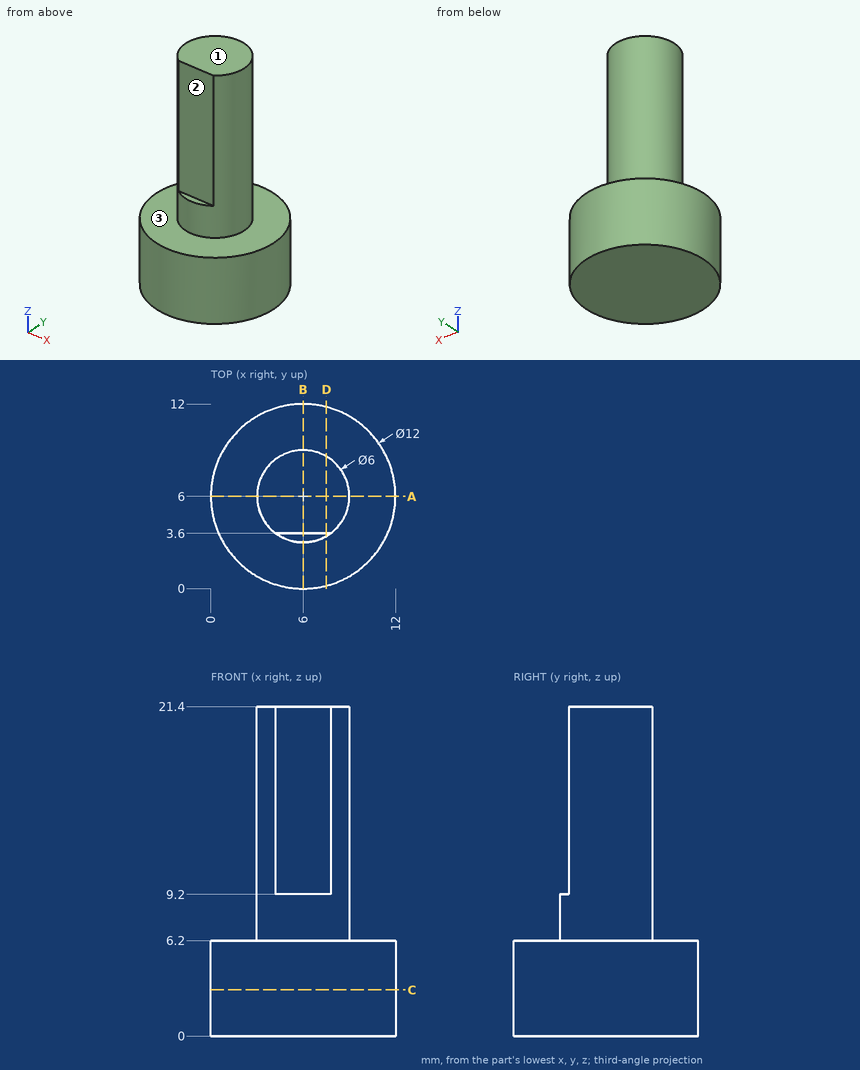
Print and shaded views of the part. All mm, measured from the part's lowest x, y and z. A direction names the side the tool comes from. Round coordinates to 2 decimals unless told otherwise and drop trailing zeros. Order: outer loops, then holes, each group sorted by start corner. A loop starts at its lowest first (then second) coordinate and runs counter-clockwise, first axis right, second up.
Q1. Slice it at A-A (y = 6). Write the cut outline in (x, z), and give its area (3 significant figures).
Q2. Slice it at B-B (x = 6). Write the cut outline in (y, z), and give its area (3 significant figures).
Q3. Slice it at D-D (x = 7.5). Write the cut outline in (y, z).
Q4. Which spindle directions (+Z, -Z, +X, -X, +Y, -Y) get a long thin tool onto all of the face, cutting with end or side? Do the marked faces 1, 2 and 3. Say none if no direction does.
Q5. Slice it at C-C (z = 3). Write the cut outline in (x, y), and give its area (3 significant figures).
Q6. Wall check: L1, parallel to Z at x = 4.75, y = 1.25; L2, parallel to X at y = 3.5, z = 4; L3, parallel to X at y = 5.5, z = 1.75. Give the ranges that are in metal, low to high.
Q7. Drop flat-ended pins along their axis: pin 1 (1.5 mm diameter, centred on x = 4.5, y = 6.5, fed in from -Z); pin 2 (6 mm diameter, centred on y = 1.5, z = 18, fed in from -X); pin 3 (1.8 mm diameter, centred on x = 5.5, z = 15, fed in from -Y); pin 4 (4 mm diameter, centred on y = 4, z = 16.5, fed in from -X). Give the stop position or say it passes through.
Results below:
1. outline: (0, 0) - (12, 0) - (12, 6.2) - (9, 6.2) - (9, 21.4) - (3, 21.4) - (3, 6.2) - (0, 6.2) - close
1. area: 166 mm2
2. outline: (0, 0) - (12, 0) - (12, 6.2) - (9, 6.2) - (9, 21.4) - (3.6, 21.4) - (3.6, 9.2) - (3, 9.2) - (3, 6.2) - (0, 6.2) - close
2. area: 158 mm2
3. outline: (0.19, 0) - (11.81, 0) - (11.81, 6.2) - (8.6, 6.2) - (8.6, 21.4) - (3.6, 21.4) - (3.6, 9.2) - (3.4, 9.2) - (3.4, 6.2) - (0.19, 6.2) - close
4. face 1: +Z, +X, -X, +Y, -Y
4. face 2: +Z, +X, -X, -Y
4. face 3: +Z
5. outline: circle Ø12 at (6, 6)
5. area: 113 mm2
6. L1: z = 0 to 6.2
6. L2: x = 0.55 to 11.45
6. L3: x = 0.02 to 11.98
7. pin 1: stops at z = 0
7. pin 2: stops at x = 3.4
7. pin 3: stops at y = 3.6
7. pin 4: stops at x = 3
